Could you check a few things on this model? Use its own coordinates, in mm. Give positions to 0.01 mm unless a question says otherwise; leave off trailing zeros. Loops run counter-clockwise (first coordinate to the right, second up) from the corner with the lowest first, then second, coordinate; pieces in that order, holes last. Notation, with made-up numbers: M 10,40 L 24,40 A30 cw 24,78 Z; hole C 52.5,46 d2. An arc over 180 degrees is marked long. Use a Markdown table: item, result. Add a question column.
1) Suppose I cut it at D-D on z = 46.5. List the corners of the cut face in (x, y) for me.
2) Suppose I cut it at C-C on x = 70.5. List the corners of the cut face in (y, z) for me, and give its area (3 significant figures).
3) If I drill on line 1 along Z through (x, y) = (0, 2.3); line 2 along Z through (x, y) = (-98.5, 2.7); line 3 along Z through (x, y) = (77.5, 1.8), over which ranges is the centre line in solid material (lowest first)? Write a range as [from, to].
4) Suppose I cut it at A-A on z = 0. List the corners of the cut face in (x, y) for me, and give its area (3 significant figures).
5) Will these pins go through, and if not, where does the flat tip stop? pin 1 Ø2.5 at (x, y) = (83.5, 3.5) entering from -Z; pin 2 Ø1.5 at (x, y) = (-83.5, 3.5) entering from +Z; pin 3 Ø3 at (x, z) = (-44.17, -25.5) entering from -Y.
6) Suppose I cut it at B-B on x = 26. List the corners of the cut face in (y, z) for me, and give its area (3 significant figures).
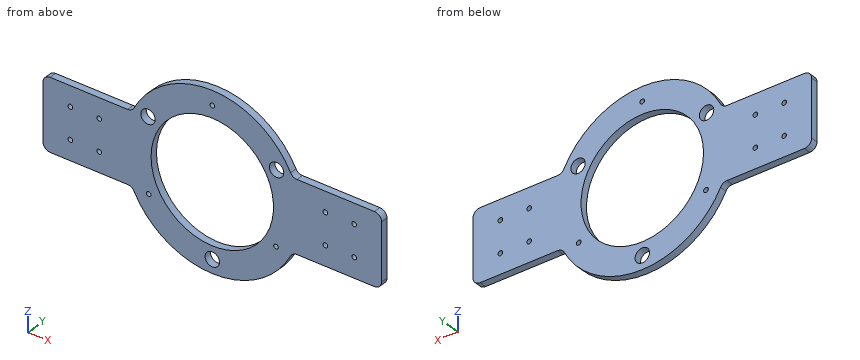
Autodesk Inventor part; units mm, degrees
ref_plane "YZ Plane" through (0, 0, 0) normal (1, 0, 0) x (0, 1, 0)
ref_plane "XZ Plane" through (0, 0, 0) normal (0, 1, 0) x (-1, 0, 0)
ref_plane "XY Plane" through (0, 0, 0) normal (0, 0, 1) x (1, 0, 0)
sketch "Sketch1" plane through (0, 0, 0) normal (0, 1, 0) x (-1, 0, 0)
  circle A0 centre (0, 0) radius 42.5
  arc A1 (55.6417, 25) -> (-55.6417, 25) centre (0, 0) ccw
  line L0 (0, 0) -> (0, -61)
  line L1 (0, 0) -> (0, 0)
  line L2 (0, 0) -> (0, -90.4875)
  line L3 (-117.5, 25) -> (-117.5, -25)
  line L4 (117.5, -25) -> (117.5, 25)
  line L5 (117.5, 25) -> (-117.5, -25) construction
  line L6 (-117.5, 25) -> (117.5, -25) construction
  line L7 (117.5, 25) -> (55.6417, 25)
  line L8 (-55.6417, 25) -> (-117.5, 25)
  line L9 (55.6417, -25) -> (117.5, -25)
  line L10 (-117.5, -25) -> (-55.6417, -25)
  arc A2 (-55.6417, -25) -> (55.6417, -25) centre (0, 0) ccw
  dimension "d0" = 85
  dimension "d29" = 61
  dimension "d46" = 235
  dimension "d47" = 50
extrude "Extrusion1" add sketch "Sketch1" along normal blind 5
sketch "Sketch2" plane through (0, 0, 0) normal (0, -1, 0) x (1, 0, 0)
  line L0 (-117.5, -25) -> (-117.5, 25)
  line L1 (-117.5, 0) -> (117.5, 0)
  line L2 (117.5, 25) -> (117.5, -25)
  arc A0 (55.6417, 25) -> (-55.6417, 25) centre (0, 0) ccw
  line L3 (0, 61) -> (0, -61)
  arc A1 (-55.6417, -25) -> (55.6417, -25) centre (0, 0) ccw
  circle A2 centre (-98.5, 11) radius 2
  line L4 (-117.5, 25) -> (-55.6417, 25)
  circle A3 centre (-78.5, 11) radius 2
  circle A4 centre (-98.5, -11) radius 2
  circle A5 centre (-78.5, -11) radius 2
  circle A6 centre (98.5, 11) radius 2
  circle A7 centre (78.5, 11) radius 2
  circle A8 centre (98.5, -11) radius 2
  circle A9 centre (78.5, -11) radius 2
  dimension "d51" = 4
  dimension "d52" = 19
  dimension "d53" = 14
  dimension "d54" = 4
  dimension "d55" = 20
hole "Hole1" at (-98.5, 0, 11) at (-78.5, 0, 11) at (-78.5, 0, -11) at (-98.5, 0, -11) at (78.5, 0, 11) at (98.5, 0, 11) at (98.5, 0, -11) at (78.5, 0, -11) direction (0, 1, 0) diameter 3.242 depth 11.8 tip angle 118
fillet "Fillet2" radius 5 8 edges at (-117.5, 2.5, -25) (-55.6417, 2.5, -25) (117.5, 2.5, -25) (55.6417, 2.5, -25) (117.5, 2.5, 25) (55.6417, 2.5, 25) (-55.6417, 2.5, 25) (-117.5, 2.5, 25)
sketch "Sketch4" plane through (0, 5, 0) normal (0, 1, 0) x (1, 0, 0)
  circle A0 centre (0, 0) radius 51.5
  point P0 (0, 51.5)
  point P1 (-44.6003, -25.75)
  point P2 (44.6003, -25.75)
  dimension "d57" = 103
  dimension "d60" = 360
hole "Pins" at (0, 5, -51.5) at (-44.6003, 5, 25.75) at (44.6003, 5, 25.75) direction (0, -1, 0) diameter 10 end through all
sketch "Sketch5" plane through (0, 5, 0) normal (0, 1, 0) x (1, 0, 0)
  circle A0 centre (0, 0) radius 51
  point P0 (0, -51)
  point P1 (0, -51)
  dimension "d69" = 102
hole "Mounting Holes" at (0, 5, 51) direction (0, -1, 0) diameter 3.242 end through all
pattern_circular "Circular Pattern1" count 3 over 360 about axis through (0, -10, 0) along (0, 1, 0) of "Mounting Holes"
properties part number "Metal Head Thing"
Answer block:
| question | item | result |
|---|---|---|
| 1 | outline | M -39.48,0 L 39.48,0 L 39.48,5 L -39.48,5 Z |
| 2 | outline | M 0,-25 L 5,-25 L 5,25 L 0,25 Z |
| 2 | area | 250 mm^2 |
| 3 | line 1 | z = [-61, -56.5], [-46.5, -42.5], [42.5, 49.38], [52.62, 61] |
| 3 | line 2 | z = [-25, -12.62], [-9.38, 9.38], [12.62, 25] |
| 3 | line 3 | z = [-25, -12.28], [-9.72, 9.72], [12.28, 25] |
| 4 | outline | M -117.5,0 L -42.5,0 L -42.5,5 L -117.5,5 Z; M 42.5,0 L 117.5,0 L 117.5,5 L 42.5,5 Z |
| 4 | area | 750 mm^2 |
| 5 | pin 1 | stops at z = -25 |
| 5 | pin 2 | stops at z = 25 |
| 5 | pin 3 | passes through |
| 6 | outline | M 0,-55.18 L 5,-55.18 L 5,-33.62 L 0,-33.62 Z; M 0,33.62 L 5,33.62 L 5,55.18 L 0,55.18 Z |
| 6 | area | 216 mm^2 |
